Here's the drawing with two shaded views (mm, measured from the low corner). I have some questions. A direction names the side the tool comes from. Round coordinates to 2 decimals unless told otherwise and drop trailing zeros. Loops run counter-clockwise (first coordinate to the right, second up) from the corner with the lowest first, then second, coordinate; pieces in that order, holes last. Notation, with made-up numbers: (-4.75, 37) - (7.25, 37) arc R13 cw to (7.25, 62) - close; hole circle Ø8 at (29.5, 79). An arc over 180 degrees is marked (long way). Use one line per item in the form item = value.
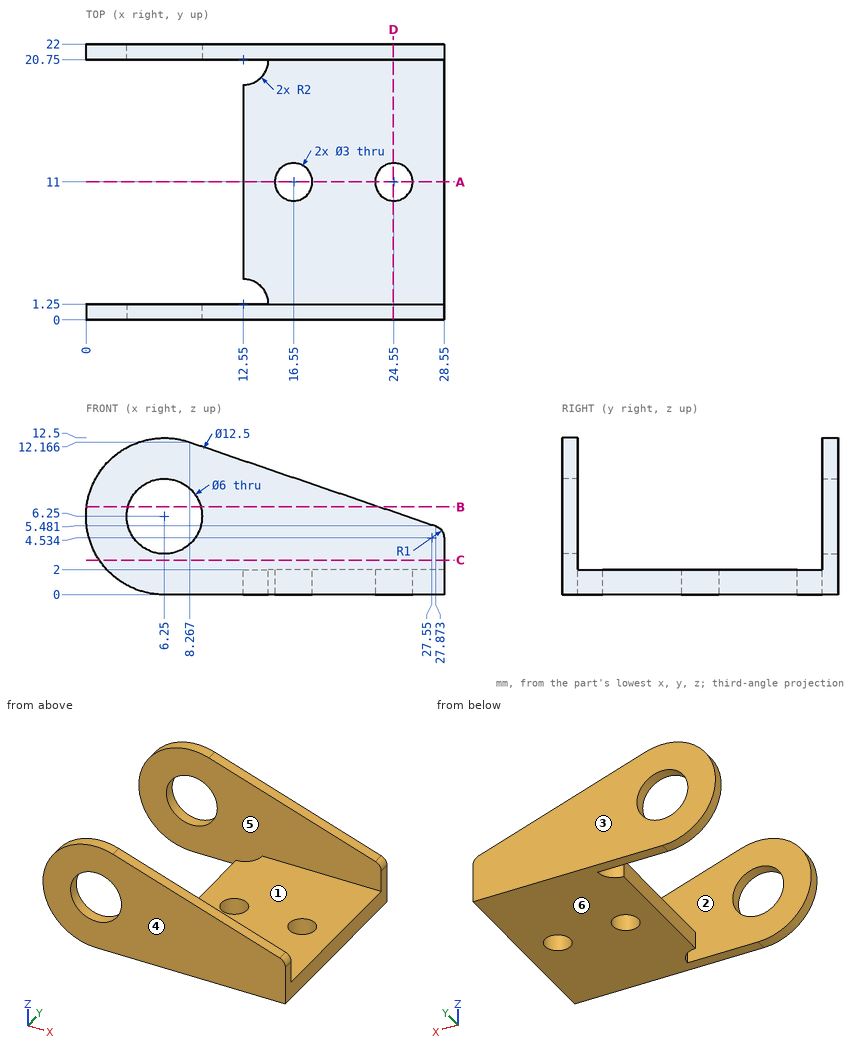
1. We'd pull the mould along Y, two halves only. Please class the marked faces 4, 5 and 6: +Y half, -Y half, draft (parallel to the pull), parting line (faces both ways), or undercut.
Solution:
face_4 = -Y half
face_5 = undercut
face_6 = draft
2. If we section it at A-A, the plane y = 11: Write out the boundary of the cut face in (x, z).
Solution:
outline = (12.55, 0) - (15.05, 0) - (15.05, 2) - (12.55, 2) - close; (18.05, 0) - (23.05, 0) - (23.05, 2) - (18.05, 2) - close; (26.05, 0) - (28.55, 0) - (28.55, 2) - (26.05, 2) - close
3. If we section it at B-B, the plane z = 7: Count the separate pieces of the cut face and the enclosed holes in it.
Solution:
separate_pieces = 4
enclosed_holes = 0
4. If we section it at D-D, the plane x = 24.5: Write out the boundary of the cut face in (y, z).
Solution:
outline = (0, 0) - (9.5, 0) - (9.5, 2) - (1.25, 2) - (1.25, 6.63) - (0, 6.63) - close; (12.5, 0) - (22, 0) - (22, 6.63) - (20.75, 6.63) - (20.75, 2) - (12.5, 2) - close
5. For P1, Ø12, axis at x = 14.5, y = 16.5, coming from the +Z side (1 decimal); P2, Ø1.5, axis at x = 20.5, y = 2.5, coming from the +Z side; P3, Ø3.5, axis at x = 6.25, z = 6.25, coming from the +Y side; P4, Ø2, axis at y = 12.5, z = 1, coming from the -X side, each with a flat end and sliding along its axis, tell me the tip position at first contact or that it passes through.
Solution:
P1 = 11.5
P2 = 2
P3 = through
P4 = 12.55
6. On a 3-axis mill with a long thin cutter (end or side, diameter ignored), from which of +Z, -Z, +X, -X, +Y, -Y can I reach the whole of each face in a straight line? I mean the marked faces 1, 2 and 3. Say none if no direction works.
Solution:
face_1 = +Z, +X, -X
face_2 = +Z, -X
face_3 = +Z, -Z, +X, -X, +Y
7. Please list where these lines run through material, in increasing order: line 1 along Y through (x, z) = (24.5, 1.5); line 2 along Y through (x, z) = (21.5, 5); line 3 along Z through (x, y) = (25, 13.5).
Solution:
line_1 = 0 to 9.5, 12.5 to 22
line_2 = 0 to 1.25, 20.75 to 22
line_3 = 0 to 2
8. If we section it at C-C, the plane z = 2.75: Write out the boundary of the cut face in (x, y).
Solution:
outline = (1.07, 0) - (28.55, 0) - (28.55, 1.25) - (1.07, 1.25) - close; (1.07, 20.75) - (28.55, 20.75) - (28.55, 22) - (1.07, 22) - close
